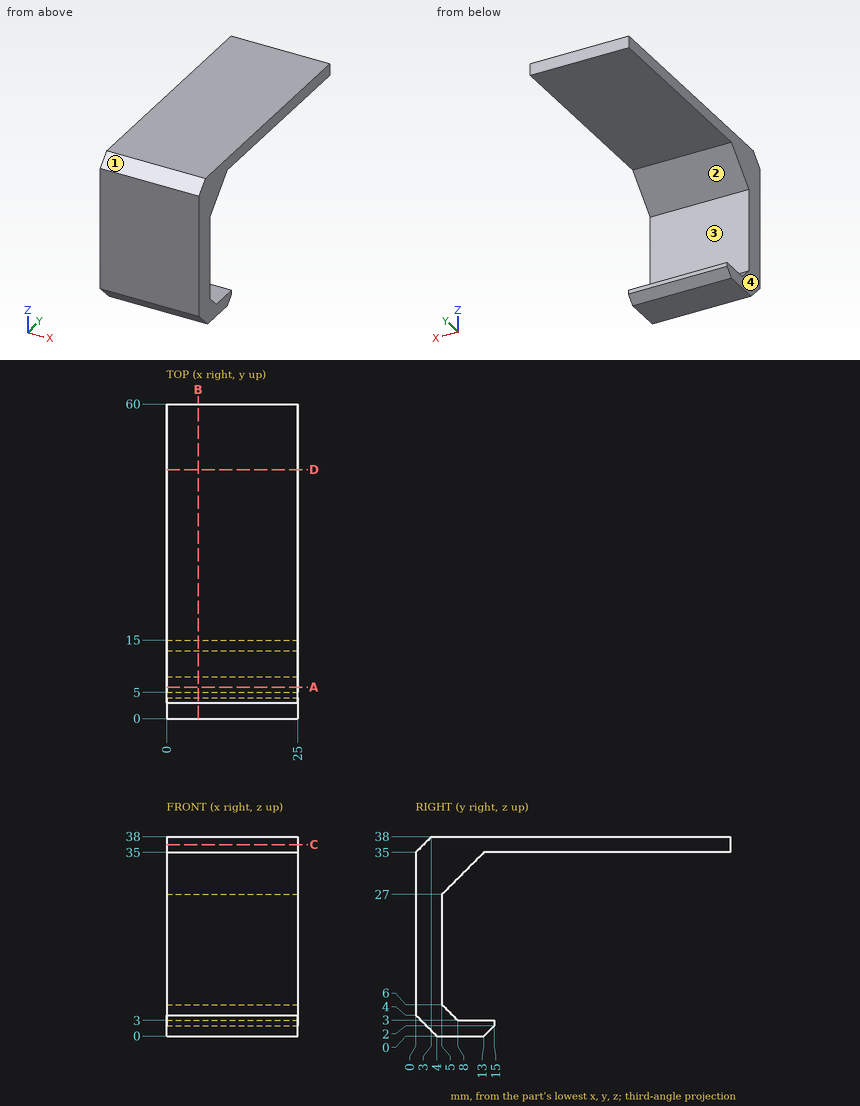
Can you work these out from the drawing? Everything is in mm from the part's minimum corner. Coordinates: 2 decimals unless noted, no trailing zeros. Write each loop counter-clockwise with the first axis right and the second up, starting at its lowest first coordinate (ties: lowest second). Pieces come first, ordered by that corner, then holes. Notation, with made-up numbers: (-31, -0.5) - (7, -0.5) arc R23 cw to (7, 30.5) - close; hole circle Ø7 at (16.25, 68.5). An arc over 180 degrees is marked (long way). Use a Markdown table: item, result.
Q1. Thinking about a two-plate mould opening in Z: for the marked faces 1, 2, 3 and 4, which applies, +Z half, -Z half, draft (parallel to the pull), parting line (faces both ways), or undercut?
Geometry check:
| item | result |
|---|---|
| face 1 | +Z half |
| face 2 | undercut |
| face 3 | undercut |
| face 4 | draft |
Q2. I'm going to push a flat-ended pin straight in: pin 1 Ø4 at (x, z) = (21, 6.5) entering from +Y. Where does the tip first touch, or does it pass through?
Geometry check:
| item | result |
|---|---|
| pin 1 | stops at y = 6.5 |
Q3. Imagine slicing it at B-B (x = 6). List the corners of the cut face in (y, z) for me.
Geometry check:
| item | result |
|---|---|
| outline | (0, 4) - (4, 0) - (13, 0) - (15, 2) - (15, 3) - (8, 3) - (5, 6) - (5, 27) - (13, 35) - (60, 35) - (60, 38) - (3, 38) - (0, 35) - close |
Q4. Imagine slicing it at D-D (y = 47.5). List the corners of the cut face in (x, z) for me, and give its area (3 significant figures).
Geometry check:
| item | result |
|---|---|
| outline | (0, 35) - (25, 35) - (25, 38) - (0, 38) - close |
| area | 75.0 mm2 |
Q5. Imagine slicing it at A-A (y = 6). List the corners of the cut face in (x, z) for me.
Geometry check:
| item | result |
|---|---|
| outline | (0, 0) - (25, 0) - (25, 5) - (0, 5) - close; (0, 28) - (25, 28) - (25, 38) - (0, 38) - close |
Q6. Please list where these lines run through material, in increasing order: L1, parallel to Z at x = 10.75, y = 13; L2, parallel to Y at x = 12.5, z = 19; L3, parallel to Y at x = 16.5, z = 30.
Geometry check:
| item | result |
|---|---|
| L1 | z = 0 to 3, 35 to 38 |
| L2 | y = 0 to 5 |
| L3 | y = 0 to 8 |
Q7. Imagine slicing it at C-C (z = 36.5). List the corners of the cut face in (x, y) for me, and give its area (3 significant figures).
Geometry check:
| item | result |
|---|---|
| outline | (0, 1.5) - (25, 1.5) - (25, 60) - (0, 60) - close |
| area | 1,460 mm2 |
